CAD build for the part. Positions are in the model's coordinates, mm. A direction names the side the tool comes from. Give positions to 0.01 mm unless a question says otherwise; leave off trailing zeros. Loops run counter-clockwise (first coordinate to the right, second up) from the corner with the lowest first, then second, coordinate; pieces in that order, holes last. Notation, with made-up numbers: M 69,33.5 L 116,33.5 A10 cw 116,43.5 Z; hole C 66,-1 d1. An arc over 180 degrees is marked long. One line per question, with ' | ' between items.
```python
from build123d import *

# Parameters (mm, degrees)
FILLET1_R   = 0.2
HEX_START   = -1.5
HEX_2_DEPTH = 1.5


with BuildPart() as part:
    # BodySke → BaseBody (revolve)
    with BuildSketch(Plane.XY, mode=Mode.PRIVATE) as basebody_sk:
        Polygon((0, 0), (0, 3.9), (0.58, 3.9), (2.48, 2), (24.61, 2), (25, 1.61), (25, 0), align=None)
    revolve(basebody_sk.sketch.rotate(Axis((0, 0, 0), (1, 0, 0)), 90), axis=Axis((0, 0, 0), (1, 0, 0)))

    # Fillet1
    fillet1_edges = [part.edges().sort_by_distance(p)[0] for p in [
        (2.48, 0, -2),
    ]]
    fillet(fillet1_edges, radius=FILLET1_R)

    # Hex 2: read off the stored shape, not the designer's step
    # Hex 2 outline → Hex 2 (cut)
    with BuildSketch(Plane.ZY.offset(HEX_START)):
        Polygon((-1.25, -0.721687836), (0, -1.443375673), (1.25, -0.721687836), (1.25, 0.721687836), (0, 1.443375673), (-1.25, 0.721687836), align=None)
    extrude(amount=HEX_2_DEPTH, mode=Mode.SUBTRACT)

    # Hex 2 2 outline → Hex 2 2 (revolve, cut)
    with BuildSketch(Plane.YX):
        Polygon((1.25, 1.5), (0, 2.221687836), (0, 1.5), align=None)
    revolve(axis=Axis((0, 0, 0), (1, 0, 0)), mode=Mode.SUBTRACT)


solid = part.part
```
Item 1: Drop flat-ended pins along their axis: P1, Ø1.6, axis at x = 1, y = 0.5, coming from the +Z side; P2, Ø1.5, axis at x = 14, y = -1, coming from the -Z side; P3, Ø0.7, axis at x = 1, y = 0, coming from the -Z side; P4, Ø4, axis at x = 19.5, y = 0, coming from the +Z side. Give the stop position or say it passes through.
Conclusion:
P1: z = 3.9 | P2: z = -1.98 | P3: z = -3.83 | P4: z = 2
Item 2: 3-axis set-ups, long thin cutter, end or side, ignore diameter. For faces 4 (the flat face through (0, 0, -2)), 5 (the flat face through (1, 0, -1.25)): which of +Z, -Z, +X, -X, +Y, -Y reach the whole face in a straight line?
Conclusion:
face 4: +Z, -Z, -X, +Y, -Y | face 5: -X
Item 3: Drill centre lines: line 1 along Y through (x, z) = (10, 0); line 2 along X through (y, z) = (2, 1); line 3 along Y through (x, z) = (15.75, 0.5). Where is each one in solid material? Low to high. Write a range as [from, to].
Conclusion:
line 1: [-2, 2] | line 2: [0, 2.24] | line 3: [-1.94, 1.94]
Item 4: Mould opens along Z. For faces 1 (the flat face through (0.76, -1.088, 0.616)), 2 (the flat face through (25, 0, 0)), 3 (the cylindrical face through (14, 2, 0)) say: pulls with the +Z half, pulls with the -Z half, needs draft (parallel to the pull), parting line crosses it, or undercut.
Conclusion:
face 1: undercut | face 2: needs draft | face 3: parting line crosses it
Item 5: Saw through at A-A on x = 7.5. Give the cut face in (y, z).
Conclusion:
outline: C 0,0 d4
